Autodesk Inventor part; units mm, degrees
ref_plane "YZ Plane" through (0, 0, 0) normal (1, 0, 0) x (0, 1, 0)
ref_plane "XZ Plane" through (0, 0, 0) normal (0, 1, 0) x (-1, 0, 0)
ref_plane "XY Plane" through (0, 0, 0) normal (0, 0, 1) x (1, 0, 0)
sketch "Sketch1" plane through (0, 0, 0) normal (0, 1, 0) x (-1, 0, 0)
  circle A0 centre (0, 0) radius 6.096
  line L0 (3.81, 0) -> (-3.81, 0) construction
  line L1 (2.5903, -2.794) -> (-2.5903, -2.794)
  line L2 (2.5903, 2.794) -> (-2.5903, 2.794)
  arc A1 (-2.5903, 2.794) -> (-2.5903, -2.794) centre (0, 0) ccw
  arc A2 (2.5903, -2.794) -> (2.5903, 2.794) centre (0, 0) ccw
  dimension "d0" = 12.192
  dimension "d2" = 5.588
  dimension "d3" = 2.794
  dimension "d13" = 3.81
  dimension "d14" = 3.81
extrude "Extrusion1" add sketch "Sketch1" along normal blind 5.08
sketch "Sketch2" plane through (0, 5.08, 0) normal (0, 1, 0) x (1, 0, 0)
  circle A0 centre (0, 0) radius 6.096
extrude "Extrusion2" add sketch "Sketch2" along normal blind 0.762
sketch "Sketch3" plane through (0, 5.842, 0) normal (0, 1, 0) x (1, 0, 0)
  arc A0 (-2.5903, 2.794) -> (-2.5903, -2.794) centre (0, 0) ccw construction
  arc A1 (-2.5903, 2.794) -> (-2.5903, -2.794) centre (0, 0) ccw
  line L0 (-2.5903, 2.794) -> (2.5903, 2.794) construction
  line L1 (-2.5903, 2.794) -> (2.5903, 2.794)
  arc A2 (2.5903, -2.794) -> (2.5903, 2.794) centre (0, 0) ccw construction
  arc A3 (2.5903, -2.794) -> (2.5903, 2.794) centre (0, 0) ccw
  line L2 (2.5903, -2.794) -> (-2.5903, -2.794) construction
  line L3 (2.5903, -2.794) -> (-2.5903, -2.794)
  arc A4 (-2.3827, 2.286) -> (-2.3827, -2.286) centre (0, 0) ccw
  line L4 (-2.3827, 2.286) -> (2.3827, 2.286)
  arc A5 (2.3827, -2.286) -> (2.3827, 2.286) centre (0, 0) ccw
  line L5 (2.3827, -2.286) -> (-2.3827, -2.286)
  point P0 (-2.5903, -2.794)
  dimension "d15" = 0.508
  dimension "d16" = 0.508
  dimension "d17" = 0.508
  dimension "d18" = 0.508
extrude "Extrusion3" add sketch "Sketch3" along normal blind 4.572 contours L4 A5 L5 A4
sketch "Sketch4" plane through (0, 10.414, 0) normal (0, 1, 0) x (1, 0, 0)
  circle A0 centre (0, 0) radius 1.524
  dimension "d10" = 3.048
extrude "Extrusion4" cut sketch "Sketch4" against normal blind 25.4
equation "\"d3\" = 0.5 * d2"
properties part number "axle extender"
Geometry: final body of the model. Coordinates: model frame, mm. A direction names the side the tool comes from. Round coordinates to 2 decimals unless told otherwise and drop trailing zeros. Write each loop counter-clockwise with the first axis right and the second up, starting at its lowest first coordinate (ties: lowest second). Pieces come first, ordered by that corner, then holes.
Item 1: Section query C-C (z = -2.5). Return loops of the section in (x, y).
Item 2: Section query A-A (y = 8.5). Return loops of the section in (x, z).
Item 3: Section query D-D (y = 2.5). Return loops of the section in (x, z), plus the area to 3 significant figures.
Item 4: Material intervals for L1, parallel to Z at x = 0, y = 7.2; L2, parallel to X at y = 8.9, z = 0; L3, parallel to Z at x = 0, y = 3, sorted ascending.
Item 5: Set-up query: faces 1 (the face through (0, 5.842, 3)), 2 (the face through (0, 3, 2.794)), 3 (the face through (0, 8, -2.286)). Return all of +Z, -Z, +X, -X, +Y, -Y with unobstructed straight access to the full face (end or side cutting, diameter ignored); none if empty.
Item 6: Pin query (flat end, axial travel): P1, Ø1, axis at x = 3, y = 7, coming from the -Z side; P2, Ø5, axis at x = -0.5, y = 8.5, coming from the +Z side; P3, Ø4, axis at y = 6, z = -3.5, coming from the -X side. Return the tip coordinate at first contact, or that it passes through.
Item 7: Mould query, pull axis X, two halves, no side actions, for faces 4 (the face through (0, 10.414, -2)), 5 (the face through (3.3, 8.1, 0)), 6 (the face through (-0.2, 7.78, -1.51)). Classes: +X half, -X half, draft (parallel to the pull), parting line (faces both ways), or undercut.
Completed:
1. outline: (-5.56, 0) - (-2.88, 0) - (-2.88, 5.08) - (2.88, 5.08) - (2.88, 0) - (5.56, 0) - (5.56, 5.84) - (-5.56, 5.84) - close
2. outline: (-2.38, -2.29) - (2.38, -2.29) arc R3.3 ccw to (2.38, 2.29) - (-2.38, 2.29) arc R3.3 ccw to start; hole circle Ø3.05 at (0, 0)
3. outline: circle Ø12.19 at (0, 0); hole (-2.59, -2.79) - (2.59, -2.79) arc R3.81 ccw to (2.59, 2.79) - (-2.59, 2.79) arc R3.81 ccw to start
3. area: 78.4 mm2
4. L1: z = -2.29 to -1.52, 1.52 to 2.29
4. L2: x = -3.3 to -1.52, 1.52 to 3.3
4. L3: z = -6.1 to -2.79, 2.79 to 6.1
5. face 1: +Y
5. face 2: -Y
5. face 3: -Z, +X, -X, +Y
6. P1: stops at z = -2.16
6. P2: stops at z = 2.29
6. P3: stops at x = -5.91
7. face 4: draft
7. face 5: +X half
7. face 6: undercut
